Here's how the part is built. I have some questions about the finished solid (model axes, mm). Round coordinates to 2 decimals unless told otherwise and drop trailing zeros. Write each loop counter-clockwise with the first axis right and the second up, starting at its lowest first coordinate (ties: lowest second). Pieces come first, ordered by that corner, then holes. Notation, with made-up numbers: (-30, 24) -> (-9, 24) arc R7 ccw to (-9, 29) -> close; hole circle Ø6 at (76.5, 57). An arc over 180 degrees is marked (long way). Answer as CSV lines item,"result".
from build123d import *

# Parameters (mm, degrees)
SKETCH1_R           = 1.55
BOSS_EXTRUDE1_DEPTH = 2


with BuildPart() as part:
    # Sketch1 → Boss-Extrude1 (new body)
    with BuildSketch(Plane(origin=(0, 0, 0), x_dir=(1, 0, 0), z_dir=(0, 1, 0))):
        with BuildLine():
            Line((-90, 90), (-90, 107))
            Line((-90, 107), (-75, 107))
            Line((-75, 107), (-75, 90))
            ThreePointArc((-75, 90), (-26.672618896, -26.672618896), (90, -75))
            Line((90, -75), (107, -75))
            Line((107, -75), (107, -90))
            Line((107, -90), (90, -90))
            ThreePointArc((90, -90), (-37.279220614, -37.279220614), (-90, 90))
        make_face()
        with Locations(Location((-82.5, 97.5, 0), (0, 0, 270))):
            Circle(SKETCH1_R, mode=Mode.SUBTRACT)
        with Locations(Location((97.5, -82.5, 0), (0, 0, 270))):
            Circle(SKETCH1_R, mode=Mode.SUBTRACT)
        with Locations(Location((-31.975919755, -31.975919755, 0), (0, 0, 270))):
            Circle(SKETCH1_R, mode=Mode.SUBTRACT)
    extrude(amount=BOSS_EXTRUDE1_DEPTH)


solid = part.part
Item 1: I need wall thicknesses on L1, parallel to Z at x = 97.5, y = 1.3; L2, parallel to X at y = 0.7, z = -97.5; L3, parallel to Z at x = 43.5, y = 0.5. Which ranges of each line are inside material? Lowest first, please.
Results found:
L1,"z = 75 to 80.95, 84.05 to 90"
L2,"x = -90 to -84.05, -80.95 to -75"
L3,"z = 68.31 to 83.89"
Item 2: Suppose I cut it at A-A, the plane y = 1.2. List the corners of the cut face in (x, z) for me.
Results found:
outline,"(-90, -107) -> (-75, -107) -> (-75, -90) arc R165 cw to (90, 75) -> (107, 75) -> (107, 90) -> (90, 90) arc R180 ccw to (-90, -90) -> close; hole circle Ø3.1 at (-82.5, -97.5); hole circle Ø3.1 at (-31.98, 31.98); hole circle Ø3.1 at (97.5, 82.5)"
Item 3: Suppose I cut it at B-B, the plane z = 53. List the corners of the cut face in (x, y) for me.
Results found:
outline,"(-19.32, 0) -> (7.68, 0) -> (7.68, 2) -> (-19.32, 2) -> close"
Item 4: Suppose I cut it at C-C, the plane x = 25.5. List the corners of the cut face in (y, z) for me, then the cut area to 3 significant figures.
Results found:
outline,"(0, 61.87) -> (2, 61.87) -> (2, 78.05) -> (0, 78.05) -> close"
area,"32.4 mm²"
Item 5: Will these pins go through, and if not, where does the flat tip stop? pin 1 (6 mm diameter, centred on x = -60, z = -34.5, fed in from +Y); pin 2 (1 mm diameter, centred on x = -21, y = 0.5, fed in from +Z); pin 3 (1 mm diameter, centred on y = 1, z = -100.5, fed in from +X).
Results found:
pin 1,"passes through"
pin 2,"stops at z = 52.09"
pin 3,"stops at x = -75"
